```python
from build123d import *

# Parameters (mm, degrees)
BOSS_EXTRUDE1_DEPTH = 30


with BuildPart() as part:
    # Sketch1 → Boss-Extrude1 (new body)
    with BuildSketch(Plane.XY):
        with BuildLine():
            Line((7.18837747, -1.206261891), (29.208382884, 21.498869199))
            Line((29.208382884, 21.498869199), (127.116350116, 21.498869199))
            Line((127.116350116, 21.498869199), (155.060416965, -19.027825416))
            Line((155.060416965, -19.027825416), (164.939583035, -12.215918359))
            Line((164.939583035, -12.215918359), (133.418209491, 33.498869199))
            Line((133.418209491, 33.498869199), (24.129802766, 33.498869199))
            Line((24.129802766, 33.498869199), (-1.425875737, 7.148056854))
            ThreePointArc((-1.425875737, 7.148056854), (-5.074472088, -5.232358113), (7.18837747, -1.206261891))
        make_face()
        Polygon((4.041451884, 0), (2.020725942, 3.5), (-2.020725942, 3.5), (-4.041451884, 0), (-2.020725942, -3.5), (2.020725942, -3.5), align=None, mode=Mode.SUBTRACT)
    extrude(amount=BOSS_EXTRUDE1_DEPTH)


solid = part.part
```
Model file for the job. Use its own axes, mm. A direction names the side the tool comes from. Round coordinates to 2 decimals unless told otherwise and drop trailing zeros. Write each loop counter-clockwise with the first axis right and the second up, starting at its lowest first coordinate (ties: lowest second). Pieces come first, ordered by that corner, then holes. Notation, with made-up numbers: (68, 57.5) - (96, 57.5) arc R16 cw to (96, 71.5) - close; hole circle Ø3 at (37, 81). An arc over 180 degrees is marked (long way). One line per item, written item: value.
(1) Two-plate mould, pull along Y, no slides. Class faces 1 (the flat face through (-3, 1.8, 14.8)), 2 (the flat face through (140.89, 1.52, 14.79)), 3 (the flat face through (80, 33.499, 15)): pulls with the +Y half, pulls with the -Y half, needs draft (parallel to the pull), parting line crosses it, or undercut.
Values follow:
face 1: undercut
face 2: pulls with the -Y half
face 3: pulls with the +Y half
(2) Cut at A-A, the plane z = 4.25. Give the cut face in (x, y), plus the area to 3 significant figures.
Values follow:
outline: (-1.43, 7.15) arc R7.29 ccw (long way) to (7.19, -1.21) - (29.21, 21.5) - (127.12, 21.5) - (155.06, -19.03) - (164.94, -12.22) - (133.42, 33.5) - (24.13, 33.5) - close; hole (-4.04, 0) - (-2.02, -3.5) - (2.02, -3.5) - (4.04, 0) - (2.02, 3.5) - (-2.02, 3.5) - close
area: 2,380 mm²
(3) 3-axis set-ups, long thin cutter, end or side, ignore diameter. For faces 4 (the flat face through (3, -1.8, 14.8)), 5 (the flat face through (18.044, 9.987, 14.79)), 6 (the flat face through (149.4, 10.32, 14.79)): which of +Z, -Z, +X, -X, +Y, -Y reach the whole face in a straight line?
Values follow:
face 4: +Z, -Z
face 5: +Z, -Z, -Y
face 6: +Z, -Z, +X, +Y
(4) Wall check: probe 1 along X at (y, z) = (-3, 4.75) (3 decimals); probe 2 along Y at (x, z) = (66.5, 25); probe 3 along X at (y, z) = (8, 17.25). Give the ranges that are in metal, low to high.
Values follow:
probe 1: x = -6.643 to -2.309, 2.309 to 6.643, 144.009 to 158.585
probe 2: y = 21.5 to 33.5
probe 3: x = -0.6 to 16.12, 136.42 to 151
(5) Cut at C-C, the plane x = 52. Give the cut face in (y, z), plus the area to 3 significant figures.
Values follow:
outline: (21.5, 0) - (33.5, 0) - (33.5, 30) - (21.5, 30) - close
area: 360 mm²
(6) Cut at B-B, the plane y = 18. Give the cut face in (x, z).
Values follow:
outline: (9.1, 0) - (25.82, 0) - (25.82, 30) - (9.1, 30) - close; (129.53, 0) - (144.11, 0) - (144.11, 30) - (129.53, 30) - close
(7) Drop flat-ended pins along their axis: P1, Ø4.5, axis at x = 0, z = 20.5, coming from the -Y side; P2, Ø3, axis at x = 0.5, z = 16.5, coming from the +Y side; P3, Ø8, axis at x = 13.5, z = 8.5, coming from the +Y side. Give the stop position or say it passes through.
Values follow:
P1: stops at y = -7.29
P2: stops at y = 10.68
P3: stops at y = 26.66
(8) Cut at D-D, the plane y = 28.5. Give the cut face in (x, z).
Values follow:
outline: (19.28, 0) - (136.87, 0) - (136.87, 30) - (19.28, 30) - close
